from build123d import *

# Parameters (mm, degrees)
BOSS_EXTRUDE1_DEPTH      = 50.8
BOSS_EXTRUDE1_DEPTH_BACK = 76.2
SKETCH1_W                = 800.1
SKETCH1_H                = 901.7
SKETCH1_W_2              = 635
SKETCH1_H_2              = 736.6
SKETCH1_3_W              = 635
SKETCH1_3_H              = 736.6
SKETCH1_3_W_2            = 584.2
SKETCH1_3_H_2            = 685.8
BOSS_EXTRUDE2_DEPTH      = 2.54
FILLET1_R                = 25.4


with BuildPart() as part:
    # Sketch1 → Boss-Extrude1 (new, two sides: drawn at the far end of the back side and taken through both)
    with BuildSketch(Plane(origin=(0, 0, 0), x_dir=(1, 0, 0), z_dir=(0, 1, 0)).offset(-BOSS_EXTRUDE1_DEPTH_BACK)):
        Rectangle(SKETCH1_W, SKETCH1_H)
        Rectangle(SKETCH1_W_2, SKETCH1_H_2, mode=Mode.SUBTRACT)
    extrude(amount=BOSS_EXTRUDE1_DEPTH + BOSS_EXTRUDE1_DEPTH_BACK)

    # Sketch1<3> → Boss-Extrude2 (add)
    with BuildSketch(Plane(origin=(0, 0, 0), x_dir=(1, 0, 0), z_dir=(0, 1, 0))):
        Rectangle(SKETCH1_3_W, SKETCH1_3_H)
        Rectangle(SKETCH1_3_W_2, SKETCH1_3_H_2, mode=Mode.SUBTRACT)
    extrude(amount=BOSS_EXTRUDE2_DEPTH)

    # Fillet1
    fillet1_edges = [part.edges().sort_by_distance(p)[0] for p in [
        (0, -76.2, 450.85),
        (-400.05, -12.7, -450.85),
        (400.05, -12.7, -450.85),
        (400.05, -76.2, 0),
        (400.05, -12.7, 450.85),
        (-400.05, -12.7, 450.85),
        (0, -76.2, -450.85),
        (-400.05, 50.8, 0),
        (0, 50.8, -450.85),
        (0, 50.8, 450.85),
        (400.05, 50.8, 0),
        (-400.05, -76.2, 0),
    ]]
    fillet(fillet1_edges, radius=FILLET1_R)


solid = part.part
Work out the finished part from the listing and answer in its coordinate system (mm). A direction names the side the tool comes from. Coordinates: 2 decimals unless noted, no trailing zeros. Order: outer loops, then holes, each group sorted by start corner. A loop starts at its lowest first (then second) coordinate and runs counter-clockwise, first axis right, second up. Notation, with made-up numbers: (29.5, -38.75) - (88.5, -38.75) arc R22 cw to (88.5, -29.75) - close; hole circle Ø4 at (-34.5, 76.25). An arc over 180 degrees is marked (long way). Put each result on its own line as item: value. Start each with the question number.
1) For faces 1 (the flat face through (-317.5, -39, 5)), 2 (the flat face through (317.5, 26, 5)), 3 (the cylindrical face through (5.25, 43.16, -443.61)), determine the directions among +Z, -Z, +X, -X, +Y, -Y from which every point of the face is accessible in a straight line to the end or side of a thin tool.
2) Find section C-C (x = -263). Give the vertices of the cut face in (y, z), plus the area to 3 significant figures.
3) Find the intervals of material crossed by line 1 (Z direction, x = -128, y = 27); line 2 (X direction, y = -42.5, z = -100.5); line 3 (Y direction, x = 113, z = -345), in increasing order. Write a range as from..to.
4) For a pull along X with two mould halves and no side action, classify faces 4 (the cylindrical face through (392, -12, 444)), 5 (the flat face through (-4, -39, -368.3)), 6 (the cylindrical face through (5.25, -68.56, 443.61)), 7 (the cylindrical face through (-392.81, -12.17, 443.21)) as released by +X, released by -X, zero draft, split by the parting line, or undercut.
5) Flat-ended cylindrical pins translate along their axes: pin 1 (3 mm diameter, centred on y = -58, z = -226.5, fed in from +X); pin 2 (14.5 mm diameter, centred on x = 142.5, y = 38.5, fed in from +Z); pin 3 (1.5 mm diameter, centred on x = -310, z = -166, fed in from -Y). Find the tip coordinate at first contact, or state that the pin passes through.
6) Find section B-B (y = -41). Give the vertices of the cut face in (x, z), plus the area to 3 significant figures.
7) Find section D-D (y = 40). Give the vertices of the cut face in (x, z), plus the area to 3 significant figures.
8) Find section A-A (z = 103). Give the vertices of the cut face in (x, y), plus the area to 3 significant figures.
Results list:
1. face 1: -Y
1. face 2: +Y
1. face 3: -Z, +X, -X, +Y
2. outline: (-76.2, -425.45) arc R25.4 ccw to (-50.8, -450.85) - (25.4, -450.85) arc R25.4 ccw to (50.8, -425.45) - (50.8, -368.3) - (2.54, -368.3) - (2.54, -342.9) - (0, -342.9) - (0, -368.3) - (-76.2, -368.3) - close; (-76.2, 368.3) - (0, 368.3) - (0, 342.9) - (2.54, 342.9) - (2.54, 368.3) - (50.8, 368.3) - (50.8, 425.45) arc R25.4 ccw to (25.4, 450.85) - (-50.8, 450.85) arc R25.4 ccw to (-76.2, 425.45) - close
2. area: 20,500 mm^2
3. line 1: z = -450.8..-368.3, 368.3..450.8
3. line 2: x = -400.05..-317.5, 317.5..400.05
3. line 3: y = 0..2.54
4. face 4: released by +X
4. face 5: undercut
4. face 6: zero draft
4. face 7: released by -X
5. pin 1: stops at x = 399.4
5. pin 2: stops at z = 450.17
5. pin 3: stops at y = 0
6. outline: (-400.05, -425.45) arc R25.4 ccw to (-374.65, -450.85) - (374.65, -450.85) arc R25.4 ccw to (400.05, -425.45) - (400.05, 425.45) arc R25.4 ccw to (374.65, 450.85) - (-374.65, 450.85) arc R25.4 ccw to (-400.05, 425.45) - close; hole (-317.5, -368.3) - (317.5, -368.3) - (317.5, 368.3) - (-317.5, 368.3) - close
6. area: 253,000 mm^2
7. outline: (-395.43, -425.45) arc R20.78 ccw to (-374.65, -446.23) - (374.65, -446.23) arc R20.78 ccw to (395.43, -425.45) - (395.43, 425.45) arc R20.78 ccw to (374.65, 446.23) - (-374.65, 446.23) arc R20.78 ccw to (-395.43, 425.45) - close; hole (-317.5, -368.3) - (317.5, -368.3) - (317.5, 368.3) - (-317.5, 368.3) - close
7. area: 238,000 mm^2
8. outline: (-400.05, -50.8) arc R25.4 ccw to (-374.65, -76.2) - (-317.5, -76.2) - (-317.5, 0) - (-292.1, 0) - (-292.1, 2.54) - (-317.5, 2.54) - (-317.5, 50.8) - (-374.65, 50.8) arc R25.4 ccw to (-400.05, 25.4) - close; (292.1, 0) - (317.5, 0) - (317.5, -76.2) - (374.65, -76.2) arc R25.4 ccw to (400.05, -50.8) - (400.05, 25.4) arc R25.4 ccw to (374.65, 50.8) - (317.5, 50.8) - (317.5, 2.54) - (292.1, 2.54) - close
8. area: 20,500 mm^2
